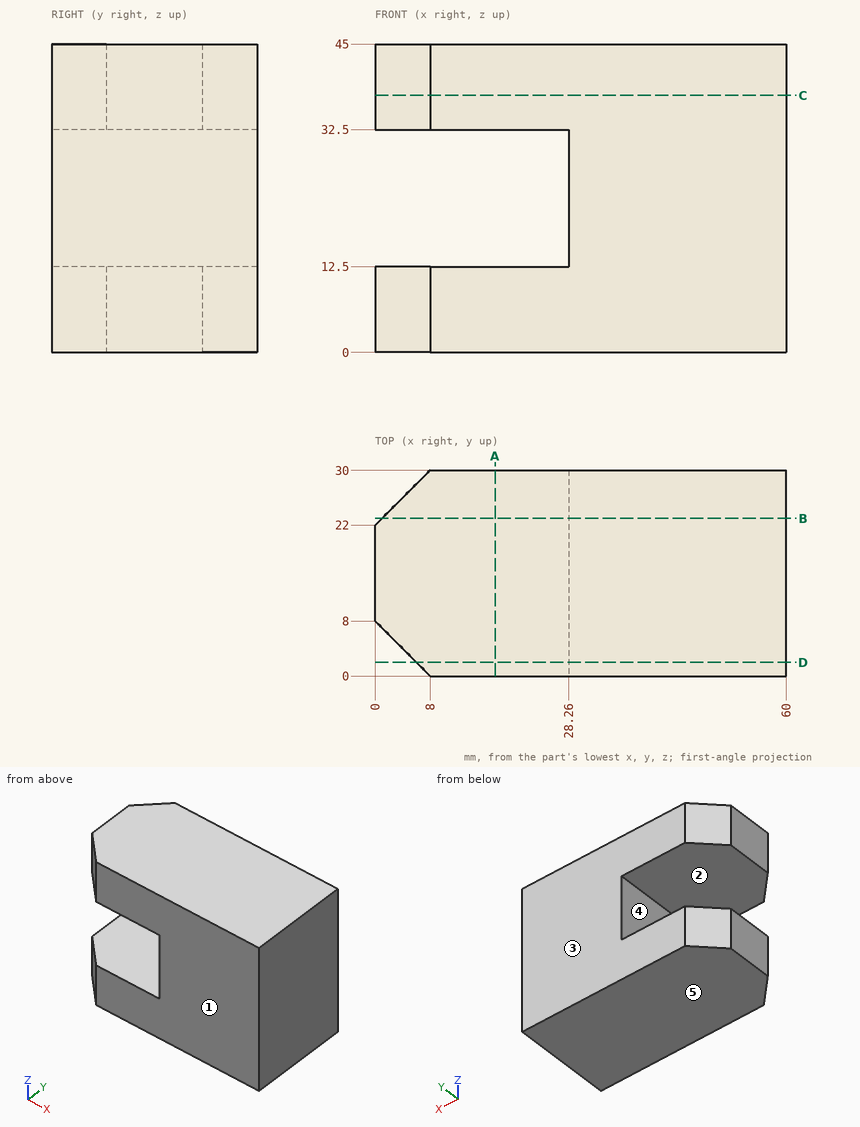
Here's the drawing with two shaded views (mm, measured from the low corner). I have some questions. A direction names the side the tool comes from. Round coordinates to 2 decimals unless told otherwise and drop trailing zeros. Loops run counter-clockwise (first coordinate to the right, second up) from the corner with the lowest first, then second, coordinate; pieces in that order, holes last. Notation, with made-up numbers: M -4,23 L 5,23 A30 ccw 5,60 Z; hole C 58,-1.5 d2. An arc over 180 degrees is marked long. Answer as a JSON object with one key per item and string values. Group by question number.
Q1. Imagine slicing it at C-C, the plane z = 37.5. Please give me the cut outline in (x, y).
Q2. Please list where these lines run through material, in increasing order: L1, parallel to Z at x = 16.5, y = 21; L2, parallel to X at y = 8.5, z = 23; L3, parallel to Y at x = 6, z = 36.
Q3. Will this pin go through, and if not, where does the flat tip stop? pin 1 (2 mm diameter, centred on y = 3.5, z = 36, fed in from -X).
Q4. Imagine slicing it at D-D, the plane y = 2. Please give me the cut outline in (x, z), then the cut area to 3 significant figures.
Q5. We'd pull the mould along Z, two halves only. Please class the marked faces 3, 4 and 5: +Z half, -Z half, draft (parallel to the pull), parting line (faces both ways), or undercut.
Q6. Imagine slicing it at A-A, the plane x = 17.5. Please give me the cut outline in (y, z).
Q7. On a 3-axis mill with a long thin cutter (end or side, diameter ignored), from which of +Z, -Z, +X, -X, +Y, -Y can I reach the whole of each face in a straight line? I mean the marked faces 1 and 2. Say none if no direction works.
Q8. Imagine slicing it at B-B, the plane y = 23. Please give me the cut outline in (x, z).
Findings:
{
 "1": {"outline": "M 0,8 L 8,0 L 60,0 L 60,30 L 8,30 L 0,22 Z"},
 "2": {"L1": "z = 0 to 12.5, 32.5 to 45", "L2": "x = 28.26 to 60", "L3": "y = 2 to 28"},
 "3": {"pin 1": "stops at x = 3.5"},
 "4": {"outline": "M 6,0 L 60,0 L 60,45 L 6,45 L 6,32.5 L 28.26,32.5 L 28.26,12.5 L 6,12.5 Z", "area": "1,980 mm2"},
 "5": {"face 3": "draft", "face 4": "undercut", "face 5": "-Z half"},
 "6": {"outline": "M 0,0 L 30,0 L 30,12.5 L 0,12.5 Z; M 0,32.5 L 30,32.5 L 30,45 L 0,45 Z"},
 "7": {"face 1": "+Z, -Z, +X, -X, -Y", "face 2": "-X, +Y, -Y"},
 "8": {"outline": "M 1,0 L 60,0 L 60,45 L 1,45 L 1,32.5 L 28.26,32.5 L 28.26,12.5 L 1,12.5 Z"}
}
